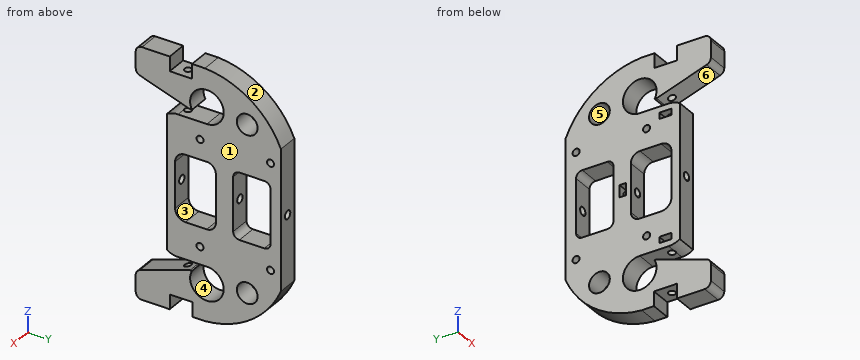
from build123d import *

# Parameters (mm, degrees)
SKETCH_1_R                = 1.7
EXTRUDE_1_DEPTH           = 10
CUT_EXTRUDE_1_DEPTH       = 67
SKETCH_3_W                = 3
SKETCH_3_H                = 5.795399196
SKETCH_3_H_2              = 5.79316294
CUT_EXTRUDE_2_DEPTH       = 8
SKETCH_5_R                = 1.7
CUT_EXTRUDE_3_DEPTH       = 31
CUT_EXTRUDE_START         = -31
SKETCH_6_R                = 1.7
CUT_EXTRUDE_4_DEPTH       = 31
SKETCH_9_R                = 5
CUT_EXTRUDE_6_DEPTH       = 10
CUT_EXTRUDE_7_DEPTH       = 10
CUT_EXTRUDE_9_DEPTH       = 10
FILLET_1_R                = 5
CUT_EXTRUDE_10_DEPTH      = 140.283882779
CUT_EXTRUDE_10_DEPTH_BACK = 10
SKETCH_12_W               = 10
SKETCH_12_H               = 11.048825586
CUT_EXTRUDE_11_DEPTH      = 7
SKETCH_14_W               = 10
SKETCH_14_H               = 10.712519762
CUT_EXTRUDE_12_DEPTH      = 7


with BuildPart() as part:
    # Эскиз1 → Бобышка-Вытянуть1 (new body)
    with BuildSketch(Plane(origin=(0, 0, 0), x_dir=(0, 0, -1), z_dir=(1, 0, 0))):
        with BuildLine():
            Line((3, 0), (10.95312335, 0))
            ThreePointArc((10.95312335, 0), (12.711116168, 0.569061652), (13.802171454, 2.060359164))
            Line((13.802171454, 2.060359164), (21.766885307, 26.20985548))
            Line((21.766885307, 26.20985548), (21.766885307, 27.126272908))
            ThreePointArc((21.766885307, 27.126272908), (11.12679914, 38.53238769), (26.145937625, 34.320931027))
            Line((26.145937625, 34.320931027), (26.145765698, 20.433139819))
            ThreePointArc((26.145765698, 20.433139819), (29.074654117, 13.361991979), (36.145765697, 10.433016021))
            Line((36.145765697, 10.433016021), (83.854234303, 10.433016021))
            ThreePointArc((83.854234303, 10.433016021), (90.925345883, 13.361991979), (93.854234302, 20.433139819))
            Line((93.854234302, 20.433139819), (93.854062375, 34.320931027))
            ThreePointArc((93.854062375, 34.320931027), (108.87320086, 38.53238769), (98.233114693, 27.126272908))
            Line((98.233114693, 27.126272908), (98.233114693, 26.20985548))
            Line((98.233114693, 26.20985548), (106.197828546, 2.060359164))
            ThreePointArc((106.197828546, 2.060359164), (107.288883832, 0.569061652), (109.04687665, 0))
            Line((109.04687665, 0), (117, 0))
            ThreePointArc((117, 0), (119.121320344, 0.878679656), (120, 3))
            Line((120, 3), (120, 67))
            ThreePointArc((120, 67), (119.121320344, 69.121320344), (117, 70))
            Line((117, 70), (3, 70))
            ThreePointArc((3, 70), (0.878679656, 69.121320344), (0, 67))
            Line((0, 67), (0, 3))
            ThreePointArc((0, 3), (0.878679656, 0.878679656), (3, 0))
        make_face()
        with Locations((34.556037496, 65)):
            Circle(SKETCH_1_R, mode=Mode.SUBTRACT)
        with Locations((34.556037496, 31)):
            Circle(SKETCH_1_R, mode=Mode.SUBTRACT)
        with Locations((85.443962504, 31)):
            Circle(SKETCH_1_R, mode=Mode.SUBTRACT)
        with Locations((85.443962504, 65)):
            Circle(SKETCH_1_R, mode=Mode.SUBTRACT)
        with BuildLine():
            Line((47, 65), (73, 65))
            ThreePointArc((73, 65), (75.121320344, 64.121320344), (76, 62))
            Line((76, 62), (76, 50))
            ThreePointArc((76, 50), (75.121320344, 47.878679656), (73, 47))
            Line((73, 47), (47, 47))
            ThreePointArc((47, 47), (44.878679656, 47.878679656), (44, 50))
            Line((44, 50), (44, 62))
            ThreePointArc((44, 62), (44.878679656, 64.121320344), (47, 65))
        make_face(mode=Mode.SUBTRACT)
        with BuildLine():
            Line((48.512942473, 38.640223749), (71.745561711, 38.640223749))
            ThreePointArc((71.745561711, 38.640223749), (76.161679417, 34.224106042), (71.745561711, 29.807988336))
            Line((71.745561711, 29.807988336), (48.512942473, 29.807988336))
            ThreePointArc((48.512942473, 29.807988336), (44.096824767, 34.224106042), (48.512942473, 38.640223749))
        make_face(mode=Mode.SUBTRACT)
    extrude(amount=EXTRUDE_1_DEPTH)

    # Эскиз2 → Вырез-Вытянуть1 (cut)
    with BuildSketch(Plane(origin=(0, 70, 0), x_dir=(1, 0, 0), z_dir=(0, 1, 0))):
        with BuildLine():
            ThreePointArc((7, 60), (6.414213562, 61.414213562), (5, 62))
            Line((5, 62), (5, 60))
            Line((5, 60), (7, 60))
        make_face()
        with BuildLine():
            Line((5, 60), (5, 62))
            ThreePointArc((5, 62), (3.585786438, 58.585786438), (7, 60))
            Line((7, 60), (5, 60))
        make_face()
    extrude(amount=-CUT_EXTRUDE_1_DEPTH, mode=Mode.SUBTRACT)

    # Эскиз3 → Вырез-Вытянуть2 (cut)
    with BuildSketch(Plane.ZY):
        with Locations((-89.477143784, 21.994873796)):
            Rectangle(SKETCH_3_W, SKETCH_3_H)
        Polygon((-62.852047751, 44.039665997), (-62.852047751, 41.024446306), (-57.047413287, 41.024446306), (-57.047413287, 44.039665997), (-59.949730519, 44.039665997), align=None)
        with Locations((-30.522856216, 21.995572621)):
            Rectangle(SKETCH_3_W, SKETCH_3_H_2)
    extrude(amount=-CUT_EXTRUDE_2_DEPTH, mode=Mode.SUBTRACT)

    # Эскиз5 → Вырез-Вытянуть3 (cut)
    with BuildSketch(Plane(origin=(0, 0, -120), x_dir=(-1, 0, 0), z_dir=(0, 0, -1))):
        with Locations(Location((-5, 22, 0), (0, 0, 292.826701249))):
            Circle(SKETCH_5_R)
    extrude(amount=-CUT_EXTRUDE_3_DEPTH, mode=Mode.SUBTRACT)

    # Эскиз6 → Вырез-Вытянуть4 (cut)
    with BuildSketch(Plane.XY.offset(CUT_EXTRUDE_START)):
        with Locations(Location((5, 22, 0), (0, 0, 247.173298751))):
            Circle(SKETCH_6_R)
    extrude(amount=CUT_EXTRUDE_4_DEPTH, mode=Mode.SUBTRACT)

    # Эскиз9 → Вырез-Вытянуть6 (cut)
    with BuildSketch(Plane.ZY):
        with Locations((-99.973969782, 53.749400687)):
            Circle(SKETCH_9_R)
        with Locations((-20.026030218, 53.749400687)):
            Circle(SKETCH_9_R)
    extrude(amount=-CUT_EXTRUDE_6_DEPTH, mode=Mode.SUBTRACT)

    # Эскиз7 → Вырез-Вытянуть7 (cut)
    with BuildSketch(Plane.ZY):
        with BuildLine():
            ThreePointArc((-71.745561711, 29.807988336), (-74.868228487, 31.101439266), (-76.161679417, 34.224106042))
            Line((-76.161679417, 34.224106042), (-76.161679417, 19))
            Line((-76.161679417, 19), (-44.096824767, 19))
            Line((-44.096824767, 19), (-44.096824767, 34.224106042))
            ThreePointArc((-44.096824767, 34.224106042), (-45.390275697, 31.101439266), (-48.512942473, 29.807988336))
            Line((-48.512942473, 29.807988336), (-71.745561711, 29.807988336))
        make_face()
    extrude(amount=-CUT_EXTRUDE_7_DEPTH, mode=Mode.SUBTRACT)

    # Эскиз10 → Вырез-Вытянуть9 (cut)
    with BuildSketch(Plane.ZY):
        Polygon((-26.82075904, 15), (-60.129252092, 15), (-92.249610227, 15), (-93.165688325, 15), (-93.165688325, 8.625567354), (-26.82075904, 8.625567354), align=None)
    extrude(amount=-CUT_EXTRUDE_9_DEPTH, mode=Mode.SUBTRACT)

    # Скругление1
    fillet_1_edges = [part.edges().sort_by_distance(p)[0] for p in [
        (5, 19, -44.096824767),
        (5, 19, -76.161679417),
    ]]
    fillet(fillet_1_edges, radius=FILLET_1_R)

    # Эскиз11 → Вырез-Вытянуть10 (cut, two sides: drawn at the far end of the back side and taken through both)
    with BuildSketch(Plane.ZY.offset(-CUT_EXTRUDE_10_DEPTH_BACK)):
        with BuildLine():
            ThreePointArc((-120.033991766, 32.77619879), (-112.271772588, 55.183752349), (-93.756122218, 70))
            Line((-93.756122218, 70), (-105.662508764, 70))
            Line((-105.662508764, 70), (-120.092282854, 70))
            Line((-120.092282854, 70), (-120.033991766, 32.77619879))
        make_face()
        with BuildLine():
            Line((0.033991766, 32.77619879), (0.092282854, 70))
            Line((0.092282854, 70), (-14.337491236, 70))
            Line((-14.337491236, 70), (-26.243877782, 70))
            ThreePointArc((-26.243877782, 70), (-7.728227412, 55.183752349), (0.033991766, 32.77619879))
        make_face()
    extrude(amount=CUT_EXTRUDE_10_DEPTH + CUT_EXTRUDE_10_DEPTH_BACK, mode=Mode.SUBTRACT)

    # Эскиз12 → Вырез-Вытянуть11 (cut)
    with BuildSketch(Plane(origin=(0, 0, -120), x_dir=(-1, 0, 0), z_dir=(0, 0, -1))):
        with Locations((-5, 21.938165939)):
            Rectangle(SKETCH_12_W, SKETCH_12_H)
    extrude(amount=-CUT_EXTRUDE_11_DEPTH, mode=Mode.SUBTRACT)

    # Эскиз14 → Вырез-Вытянуть12 (cut)
    with BuildSketch(Plane.XY):
        with Locations((5, 21.770013027)):
            Rectangle(SKETCH_14_W, SKETCH_14_H)
    extrude(amount=-CUT_EXTRUDE_12_DEPTH, mode=Mode.SUBTRACT)


solid = part.part
Here's how the part is built. I have some questions about the finished solid (model axes, mm). Face numbers are marked on the shaded views. A direction names the side the tool comes from. Coordinates: 2 decimals unless noted, no trailing zeros. Loops run counter-clockwise (first coordinate to the right, second up) from the corner with the lowest first, then second, coordinate; pieces in that order, holes last.
1. Imagine slicing it at A-A, the plane y = 31. Please give me the cut outline in (x, z).
2. For P1, Ø3, axis at x = 5.5, y = 54, coming from the -Z side; P2, Ø2.5, axis at x = 3.5, y = 42.5, coming from the +Z side; P3, Ø1.7, axis at x = 4.5, y = 21.5, coming from the -Z side, each with a flat end and sliding along its axis, tell me the tip position at first contact or that it passes through.
3. If we mould it in two halves opening along Z, with no side actions, what happens to the marked faces 1, 2, 3 and 4? For each: pulls with the +Z half, pulls with the -Z half, needs draft (parallel to the pull), parting line crosses it, or undercut.
4. Imagine slicing it at C-C, the plane y = 60. Please give me the cut outline in (x, z), and give its area (3 significant figures).
5. For the marked faces 5 and 6, which set-ups out of +Z, -Z, +X, -X, +Y, -Y let a thin tool reach every point of the face, with its end or its side?
6. I need wall thicknesses on L1, parallel to Y at x = 7, z = -69; L2, parallel to Z at x = 6, y = 30; L3, parallel to Z at x = 7, y = 37.5. Which ranges of each line are inside material? Lowest first, please.
7. Imagine slicing it at B-B, the plane z = -86. Please give me the cut outline in (x, y).
Taken from the geometry:
1. outline: (0, -120) - (10, -120) - (10, -109.34) - (0, -109.34) - close; (0, -93.85) - (10, -93.85) - (10, -87.14) - (0, -87.14) - close; (0, -83.74) - (10, -83.74) - (10, -76.16) - (0, -76.16) - close; (0, -44.1) - (10, -44.1) - (10, -36.26) - (0, -36.26) - close; (0, -32.86) - (10, -32.86) - (10, -26.15) - (0, -26.15) - close; (0, -10.66) - (10, -10.66) - (10, 0) - (0, 0) - close
2. P1: stops at z = -114.02
2. P2: stops at z = -1.27
2. P3: stops at z = -87.98
3. face 1: needs draft
3. face 2: pulls with the +Z half
3. face 3: undercut
3. face 4: undercut
4. outline: (0, -108.32) - (10, -108.32) - (10, -76) - (0, -76) - close; (0, -44) - (10, -44) - (10, -11.68) - (0, -11.68) - close
4. area: 646 mm2
5. face 5: +X, -X
5. face 6: +X, -X, -Y
6. L1: y = 15 to 19, 38.64 to 47, 65 to 70
6. L2: z = -120 to -108.81, -93.85 to -86.82, -84.07 to -76.16, -44.1 to -35.93, -33.18 to -26.15, -11.19 to 0
6. L3: z = -119.52 to -109.4, -94.5 to -74.71, -45.55 to -25.5, -10.6 to -0.48
7. outline: (0, 15) - (10, 15) - (10, 29.39) - (0, 29.39) - close; (0, 32.61) - (10, 32.61) - (10, 63.39) - (0, 63.39) - close; (0, 66.61) - (10, 66.61) - (10, 70) - (0, 70) - close
